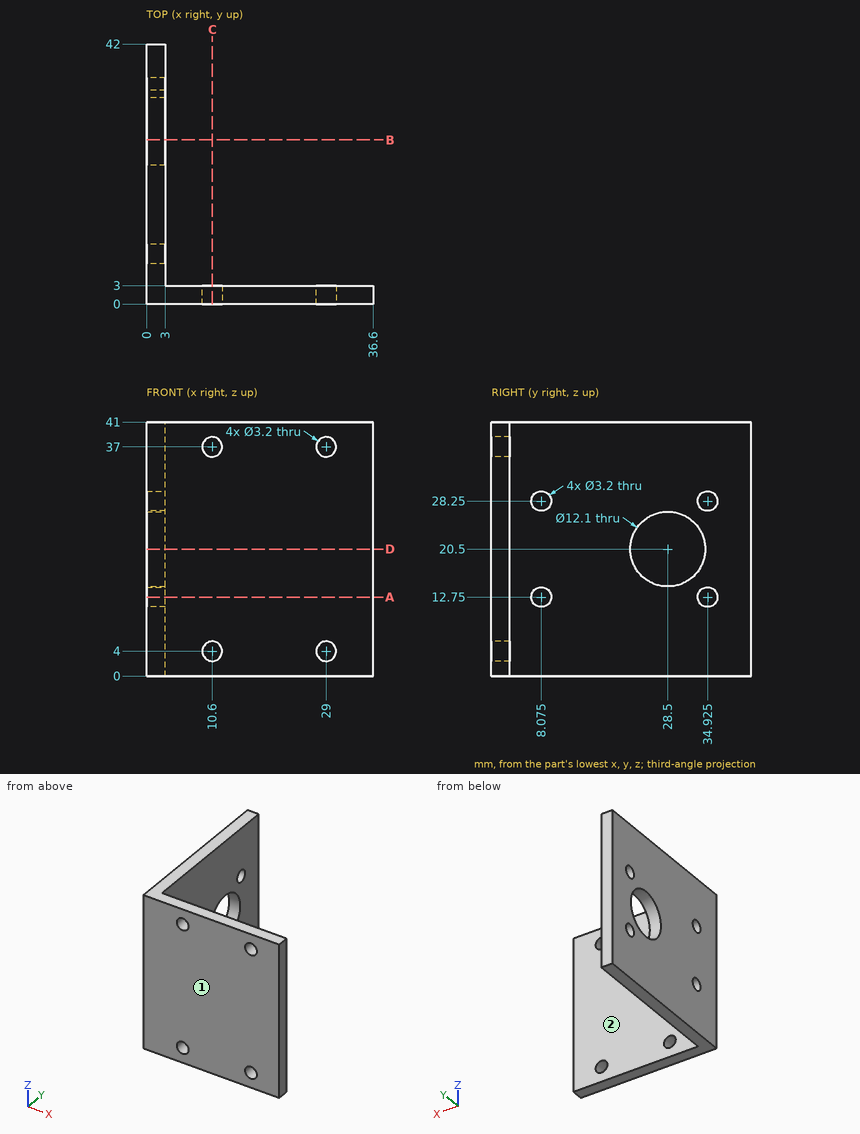
Design review of the part shown in the three views and the two pictorial views. Dimensions are in mm from the part's minimum x, y and z. A direction names the side the tool comes from. Coordinates: 2 decimals unless noted, no trailing zeros. Write each loop counter-clockwise with the first axis right and the second up, starting at its lowest first coordinate (ties: lowest second). Pieces come first, ordered by that corner, then holes. Notation, with made-up numbers: (13.5, 13) - (19.5, 13) arc R15 ccw to (19.5, 21) - close; hole circle Ø3 at (45, 82.25). An arc over 180 degrees is marked (long way). Write item = value, one per line.
(1) For line 1 (X direction, y = 0.6, z = 37); line 2 (Y direction, x = 1.35, z = 20.5); line 3 (Y direction, x = 27, z = 33.5), list the stretches that pass through material, from the lowest coordinate up. Write a range as [from, to].
Result sheet:
line_1 = [0, 9], [12.2, 27.4], [30.6, 36.6]
line_2 = [0, 22.45], [34.55, 42]
line_3 = [0, 3]
(2) Machinability: for the marked faces 1 and 2, which of the approach directions +Z, -Z, +X, -X, +Y, -Y give a long, thin tool a straight path to every point of the face, cutting with its end or side? Answer none if there is none.
Result sheet:
face_1 = +Z, -Z, +X, -X, -Y
face_2 = +Z, -Z, +X, +Y
(3) Consider section B-B, the plane y = 26.5. Give the boundary of the cut face in (x, z).
Result sheet:
outline = (0, 0) - (3, 0) - (3, 14.79) - (0, 14.79) - close; (0, 26.21) - (3, 26.21) - (3, 41) - (0, 41) - close
(4) Consider section D-D, the plane z = 20.5. Give the boundary of the cut face in (x, y), then the cut area to 4 significant figures.
Result sheet:
outline = (0, 0) - (36.6, 0) - (36.6, 3) - (3, 3) - (3, 22.45) - (0, 22.45) - close; (0, 34.55) - (3, 34.55) - (3, 42) - (0, 42) - close
area = 190.5 mm^2
(5) Consider section C-C, the plane x = 10.6. Give the boundary of the cut face in (y, z), then the cut area to 3 significant figures.
Result sheet:
outline = (0, 0) - (3, 0) - (3, 2.4) - (0, 2.4) - close; (0, 5.6) - (3, 5.6) - (3, 35.4) - (0, 35.4) - close; (0, 38.6) - (3, 38.6) - (3, 41) - (0, 41) - close
area = 104 mm^2
(6) For P1, Ø3.5, axis at x = 10.6, z = 37, coming from the +Y side; P2, Ø19.5, axis at y = 28.5, z = 20.5, coming from the +X side, all flat-tipped, find the tip position at first contact; note any pin that passes through.
Result sheet:
P1 = 3
P2 = 3
(7) Consider section A-A, the plane z = 12.75. Give the boundary of the cut face in (x, y) (3 decimals).
Result sheet:
outline = (0, 0) - (36.6, 0) - (36.6, 3) - (3, 3) - (3, 6.475) - (0, 6.475) - close; (0, 9.675) - (3, 9.675) - (3, 33.325) - (0, 33.325) - close; (0, 36.525) - (3, 36.525) - (3, 42) - (0, 42) - close
